For this review, take the finished solid that the model builds, in its own axes (mm). A direction names the side the tool comes from. Give positions to 0.01 mm unless a question says otherwise; leave off trailing zeros. Write each loop counter-clockwise with the first axis right and the second up, starting at its lowest first coordinate (ties: lowest second). Pieces come first, ordered by that corner, then holes.
Q1. We need section B-B (y = 38.1). Write out the cut boundary in (x, z), then the cut area to 3 significant figures.
Q2. Insertion check: P1, Ø4.5, axis at x = 6.35, z = -31.75, coming from the -Y side; P2, Ø5.5, axis at y = 38.1, z = -106.36, coming from the +X side. Each pin has a flat end and moves straight along its axis. Give the tip position at first contact, or say it passes through.
Q3. We need section C-C (x = 5). Give the number of separate pieces and of enclosed holes in the cut face, then the cut area to 3 significant figures.
Q4. We need section A-A (y = 12.7). Write out the cut boundary in (x, z), then the cut area to 3 significant figures.
Q5. Mouldability with a two-part tool opening along Z and no side actions: class faces 3 (the flat face through (6, 26, -114.3)), 4 (the flat face through (6, 25, 0)), 5 (the flat face through (12.7, 25, -56)), 6 (the cylindrical face through (6.44, 18.9, -9.31)) as released by +Z, released by -Z, zero draft, split by the parting line, or undercut.
Q6. Machinability: for faces 1 (the cylindrical face through (6.241, 9.658, -29.263)), 2 (the flat face through (6, 50.8, -56)), which of the approach directions +Z, -Z, +X, -X, +Y, -Y give a long, thin tool a straight path to every point of the face, cutting with its end or side? Answer none if there is none.
Q7. For line 1 (Z direction, x = 6.35, y = 4.75); line 2 (Z direction, x = 6.35, y = 10.5); line 3 (Z direction, x = 4.75, y = 14), list the stretches that pass through material, from the lowest coordinate up.
Autodesk Inventor part; units mm, degrees
ref_plane "YZ Plane" through (0, 0, 0) normal (1, 0, 0) x (0, 1, 0)
ref_plane "XZ Plane" through (0, 0, 0) normal (0, 1, 0) x (-1, 0, 0)
ref_plane "XY Plane" through (0, 0, 0) normal (0, 0, 1) x (1, 0, 0)
sketch "Sketch2" plane through (0, 0, 0) normal (1, 0, 0) x (0, 1, 0)
  line L0 (0, 0) -> (50.8, 0)
  line L1 (50.8, 0) -> (50.8, -114.3)
  line L2 (50.8, -114.3) -> (0, -114.3)
  line L3 (0, -114.3) -> (0, 0)
  circle A0 centre (12.7, -7.9375) radius 6.35
  point P0 (38.1, -106.3625)
  dimension "d0" = 50.8
  dimension "d1" = 114.3
  dimension "d2" = 98.425
  dimension "d3" = 25.4
  dimension "d4" = 12.7
  dimension "d5" = 7.9375
  dimension "d15" = 12.7
extrude "Extrusion1" add sketch "Sketch2" along normal blind 12.7 contours L0 L1 L2 L3 | A0
hole "Hole1" at (0, 38.1, -106.3625) direction (1, 0, 0) diameter 6.35 depth 19.05 tip angle 118
hole "Hole2" at (0, 12.7, -7.9375) direction (1, 0, 0) diameter 12.7 depth 19.05 tip angle 118
sketch "Sketch3" plane through (0, 0, -114.3) normal (0, -1, 0) x (1, 0, 0)
  line L0 (0, 114.3) -> (0, 0)
  line L1 (0, 0) -> (12.7, 0)
  line L2 (12.7, 114.3) -> (12.7, 0)
  line L3 (0, 114.3) -> (12.7, 114.3)
  line L4 (0, 114.3) -> (0, 0)
  line L5 (0, 0) -> (12.7, 0)
  line L6 (12.7, 114.3) -> (12.7, 0)
  line L7 (0, 114.3) -> (12.7, 114.3)
  point P0 (6.35, 82.55)
  point P1 (6.35, 19.05)
  dimension "d23" = 63.5
  dimension "d24" = 19.05
hole "Hole3" at (6.35, 0, -31.75) at (6.35, 0, -95.25) direction (0, 1, 0) diameter 4.9784 depth 19.05 tip angle 118
properties part number "clolecton wheel holder"
Computed:
1. outline: (0, -114.3) - (12.7, -114.3) - (12.7, -109.54) - (0, -109.54) - close; (0, -103.19) - (12.7, -103.19) - (12.7, 0) - (0, 0) - close
1. area: 1,370 mm2
2. P1: stops at y = 19.19
2. P2: passes through
3. separate pieces: 1
3. enclosed holes: 2
3. area: 5,490 mm2
4. outline: (0, -114.3) - (12.7, -114.3) - (12.7, -14.29) - (0, -14.29) - close; (0, -1.59) - (12.7, -1.59) - (12.7, 0) - (0, 0) - close; hole circle Ø4.98 at (6.35, -95.25); hole circle Ø4.98 at (6.35, -31.75)
4. area: 1,250 mm2
5. face 3: released by -Z
5. face 4: released by +Z
5. face 5: zero draft
5. face 6: undercut
6. face 1: -Y
6. face 2: +Z, -Z, +X, -X, +Y
7. line 1: z = -114.3 to -97.74, -92.76 to -34.24, -29.26 to 0
7. line 2: z = -114.3 to -97.74, -92.76 to -34.24, -29.26 to -13.89, -1.98 to 0
7. line 3: z = -114.3 to -97.16, -93.34 to -33.66, -29.84 to -14.15, -1.72 to 0
